from build123d import *

# Parameters (mm, degrees)
IZIM1_W                     = 750
IZIM1_H                     = 80
IZIM1_R                     = 5
Y_KSEKLIK_EKSTR_ZYON1_DEPTH = 30
KES_EKSTR_ZYON1_DEPTH       = 600


with BuildPart() as part:
    # Çizim1 → Yükseklik-Ekstrüzyon1 (new body)
    with BuildSketch(Plane(origin=(0, 0, 0), x_dir=(1, 0, 0), z_dir=(0, 1, 0))):
        Rectangle(IZIM1_W, IZIM1_H)
        with Locations((-300, 0)):
            Circle(IZIM1_R, mode=Mode.SUBTRACT)
        with Locations((-225, 0)):
            Circle(IZIM1_R, mode=Mode.SUBTRACT)
    extrude(amount=-Y_KSEKLIK_EKSTR_ZYON1_DEPTH)

    # Çizim3 → Kes-Ekstrüzyon1 (cut)
    with BuildSketch(Plane.ZY.offset(375)):
        Polygon((-30, -30), (-30, -15), (30, -15), (30, -30), (40, -30), (40, 0), (-40, 0), (-40, -30), align=None)
    extrude(amount=-KES_EKSTR_ZYON1_DEPTH, mode=Mode.SUBTRACT)


solid = part.part
Design review of the part built by this model. Coordinates are the model's own, in mm. A direction names the side the tool comes from. Round coordinates to 2 decimals unless told otherwise and drop trailing zeros. Loops run counter-clockwise (first coordinate to the right, second up) from the corner with the lowest first, then second, coordinate; pieces in that order, holes last. Notation, with made-up numbers: (-31, -35.5) -> (-19, -35.5) arc R32 ccw to (-19, -8.5) -> close; hole circle Ø3 at (66, 40). An arc over 180 degrees is marked (long way). Use one line per item in the form item = value. Start each with the question number.
Q1. We need section C-C on x = -189.5. Give the boundary of the cut face in (y, z).
Q2. For pin 1 Ø16 at (x, z) = (-300, 0) entering from +Y; pin 2 Ø7.5 at (x, y) = (-116, -22.5) entering from -Z; pin 3 Ø7.5 at (x, y) = (5, -21) entering from +Z, all flat-tipped, find the tip position at first contact; note any pin that passes through.
Q3. Machinability: for faces 1 (the face through (-79, -15, 0)), 2 (the face through (-79, -22, 30)), 3 (the face through (-79, -23, -30)), which of the approach directions +Z, -Z, +X, -X, +Y, -Y give a long, thin tool a straight path to every point of the face, cutting with its end or side? Answer none if there is none.
Q4. Wall thickness on line 1 along X through (y, z) = (-23.5, 0); line 2 along Z through (x, y) = (-225, -23.75); line 3 along Z through (x, y) = (214, -24.5): over which ranges is each line inside the solid? List them lowest first. Write a range as [from, to].
Q5. We need section B-B on z = 12. Give the boundary of the cut face in (x, y), then the cut area to 3 significant figures.
Q6. We need section A-A on y = -21.25. Give the boundary of the cut face in (x, z), then the cut area to 3 significant figures.
Calculated:
q1.outline = (-30, -30) -> (-15, -30) -> (-15, 30) -> (-30, 30) -> close
q2.pin_1 = -15
q2.pin_2 = -30
q2.pin_3 = 30
q3.face_1 = +Z, -Z, -X, +Y
q3.face_2 = +Z, -X, +Y, -Y
q3.face_3 = -Z, -X, +Y, -Y
q4.line_1 = [-375, -305], [-295, -230], [-220, 375]
q4.line_2 = [-30, -5], [5, 30]
q4.line_3 = [-30, 30]
q5.outline = (-375, -30) -> (375, -30) -> (375, 0) -> (225, 0) -> (225, -15) -> (-375, -15) -> close
q5.area = 13,500 mm²
q6.outline = (-375, -30) -> (225, -30) -> (225, -40) -> (375, -40) -> (375, 40) -> (225, 40) -> (225, 30) -> (-375, 30) -> close; hole circle Ø10 at (-300, 0); hole circle Ø10 at (-225, 0)
q6.area = 47,800 mm²
